Geometry: final body of the model. Coordinates: model frame, mm. A direction names the side the tool comes from. Round coordinates to 2 decimals unless told otherwise and drop trailing zeros. Loops run counter-clockwise (first coordinate to the right, second up) from the corner with the lowest first, then second, coordinate; pieces in that order, holes last. Notation, with made-up numbers: M 61.5,-33 L 109.5,-33 A34 ccw 109.5,6 Z; hole C 35,53 d6. An arc over 180 degrees is marked long. Answer as a JSON object with one key per item and string values.
from build123d import *

# Parameters (mm, degrees)
F0_W      = 10
F0_H      = 36
F0_H_2    = 10
F0_W_2    = 58
F0_H_3    = 48
F1_DEPTH  = 50
F4_DEPTH  = 58.001
F2_R      = 8
F5_DEPTH  = 25
F6_R      = 15
F7_R      = 5
F9_DEPTH  = 5
F10_R     = 25
F13_DEPTH = 25
F12_R     = 9
F14_DEPTH = 25
F15_DEPTH = 25


# Not quite as in the source:
# - after a boolean that leaves OpenCascade's solid faulty, fix() repairs it


with BuildPart() as f1:
    # F0 (on Front) → F1 (new body, symmetric)
    with BuildSketch(Plane.XZ):
        with Locations((5, 28)):
            Rectangle(F0_W, F0_H)
        with Locations((5, 5)):
            Rectangle(F0_W, F0_H_2)
        with Locations((39, 5)):
            Rectangle(F0_W_2, F0_H_2)
        with Locations((73, 5)):
            Rectangle(F0_W, F0_H_2)
        with Locations((73, -24)):
            Rectangle(F0_W, F0_H_3)
    extrude(amount=F1_DEPTH, both=True)

    # F3 (on face) → F4 (cut, through all)
    with BuildSketch(Plane.XY.offset(10)):
        with BuildLine():
            Line((78, -19), (40, -19))
            ThreePointArc((40, -19), (18.7867965644, -27.7867965644), (10, -49))
            Line((10, -49), (10, -50))
            Line((10, -50), (78, -50))
            Line((78, -50), (78, -19))
        make_face()
        with BuildLine():
            ThreePointArc((10, 49), (18.7867965644, 27.7867965644), (40, 19))
            Line((40, 19), (78, 19))
            Line((78, 19), (78, 50))
            Line((78, 50), (10, 50))
            Line((10, 50), (10, 49))
        make_face()
    extrude(amount=-F4_DEPTH, mode=Mode.SUBTRACT)

    # F2 (on face) → F5 (cut)
    with BuildSketch(Plane.YZ.offset(10)):
        with Locations((30, 28)):
            Circle(F2_R)
        with Locations((-30, 28)):
            Circle(F2_R)
    extrude(amount=-F5_DEPTH, mode=Mode.SUBTRACT)

    # F6
    f6_edges = [f1.edges().sort_by_distance(p)[0] for p in [
        (78, 0, 10),
    ]]
    fillet(f6_edges, radius=F6_R)

    # F7
    f7_edges = [f1.edges().sort_by_distance(p)[0] for p in [
        (68, 0, 0),
    ]]
    fillet(f7_edges, radius=F7_R)

    # F8 (on Front) → F9 (join, symmetric)
    with BuildSketch(Plane.XZ):
        with BuildLine():
            ThreePointArc((35, 20), (17.3223304703, 27.3223304703), (10, 45))
            Line((10, 45), (10, 10))
            Line((10, 10), (40, 10))
            Line((40, 10), (63, 10))
            ThreePointArc((63, 10), (73.6066017178, 5.6066017178), (78, -5))
            Line((78, -5), (78, -48))
            Line((78, -48), (88, -48))
            Line((88, -48), (88, 20))
            Line((88, 20), (35, 20))
        make_face()
    extrude(amount=F9_DEPTH, both=True)

    # F10
    f10_edges = [f1.edges().sort_by_distance(p)[0] for p in [
        (88, 0, 20),
    ]]
    fillet(f10_edges, radius=F10_R)

    # F12 (on offset) → F13 (cut)
    with BuildSketch(Plane.YZ.offset(90)):
        with BuildLine():
            ThreePointArc((0, -48), (-13.4350288425, -42.4350288425), (-19, -29))
            Line((-19, -29), (-19, -48))
            Line((-19, -48), (-5, -48))
            Line((-5, -48), (0, -48))
        make_face()
        with BuildLine():
            Line((19, -48), (19, -29))
            ThreePointArc((19, -29), (13.4350288425, -42.4350288425), (0, -48))
            Line((0, -48), (5, -48))
            Line((5, -48), (19, -48))
        make_face()
    extrude(amount=-F13_DEPTH, mode=Mode.SUBTRACT)

    # F12 (on offset) → F14 (join)
    with BuildSketch(Plane.YZ.offset(90)):
        with BuildLine():
            ThreePointArc((0, -48), (13.4350288425, -42.4350288425), (19, -29))
            ThreePointArc((19, -29), (0, -10), (-19, -29))
            ThreePointArc((-19, -29), (-13.4350288425, -42.4350288425), (0, -48))
        make_face()
        with Locations((0, -29)):
            Circle(F12_R, mode=Mode.SUBTRACT)
    extrude(amount=-F14_DEPTH)

    add(f1.part.fix(), mode=Mode.REPLACE)

    # F12 (on offset) → F15 (cut)
    with BuildSketch(Plane.YZ.offset(90)):
        with Locations((0, -29)):
            Circle(F12_R)
    extrude(amount=-F15_DEPTH, mode=Mode.SUBTRACT)


solid = f1.part
1) Section query C-C (x = 71). Return the cut outline in (y, z), and give its area (3 significant figures).
Results:
{"outline": "M -19,-29 A19 ccw 19,-29 L 19,7.69 L 5,7.69 L 5,18.69 L -5,18.69 L -5,7.69 L -19,7.69 Z; hole C 0,-29 d18", "area": "1,820 mm2"}
2) Pin query (flat end, axial travel): P1, Ø10, axis at x = 34, y = 18.5, coming from the -Z side; P2, Ø19, axis at y = 5, z = -19, coming from the -X side; P3, Ø4, axis at x = 69, y = -19, coming from the -Z side. Return the tip coordinate at first contact, or that it passes through.
Results:
{"P1": "z = 0", "P2": "x = 65", "P3": "z = -37.49"}
3) Section query A-A (y = -1.5). Return the cut outline in (x, z), and give its area (3 significant figures).
Results:
{"outline": "M 0,0 L 63,0 A5 cw 68,-5 L 68,-10.06 L 65,-10.06 L 65,-20.13 L 90,-20.13 L 90,-10.06 L 88,-10.06 L 88,-5 A25 ccw 63,20 L 35,20 A25 cw 10,45 L 10,46 L 0,46 Z; M 65,-47.94 L 90,-47.94 L 90,-37.87 L 65,-37.87 Z", "area": "2,730 mm2"}
4) Reachability of faces 1 (the flat face through (65, -4.5, -37.2)), 2 (the flat face through (78, -14, -12)), 3 (the cylindrical face through (73.49, 11.9, 5.72)) from +Z, -Z, +X, -X, +Y, -Y: full face, straight path, thin tool, end or side. Return the list, or none.
Results:
{"face 1": "-Z, -X, +Y, -Y", "face 2": "+Z, +X, -Y", "face 3": "+Z, +X, +Y"}
5) Ray query, line 1 (Y direction, x = 78, z = -29); line 2 (Z direction, x = 4.5, y = -30); line 3 (X direction, y = -41, z = 39). Return the intervals inside material, ascending.
Results:
{"line 1": "-19 to -9, 9 to 19", "line 2": "0 to 20, 36 to 46", "line 3": "0 to 10"}
6) Section query D-D (z = 28). Return the cut outline in (x, y), and give its area (3 significant figures).
Results:
{"outline": "M 0,-50 L 10,-50 L 10,-38 L 0,-38 Z; M 0,-22 L 10,-22 L 10,-5 L 16.67,-5 L 16.67,5 L 10,5 L 10,22 L 0,22 Z; M 0,38 L 10,38 L 10,50 L 0,50 Z", "area": "747 mm2"}
7) Pull-direction query (Z, two-part tool) for faces 4 (the flat face through (31, 12, 10)), 5 (the flat face through (0, -1, 23)), 6 (the flat face through (68, 0, -9)); classes: +Z half, -Z half, draft (parallel to the pull), parting line (faces both ways), or undercut.
Results:
{"face 4": "+Z half", "face 5": "draft", "face 6": "undercut"}
8) Section query B-B (x = 54). Return the cut outline in (y, z).
Results:
{"outline": "M -19,0 L 19,0 L 19,10 L 5,10 L 5,20 L -5,20 L -5,10 L -19,10 Z"}
